from build123d import *

# Parameters (mm, degrees)
SKETCH1_R                        = 4
BOSS_EXTRUDE1_DEPTH              = 90
CHAMFER1_SIZE                    = 0.6
CUT_EXTRUDE1_START               = -1.4
SKETCH2_R                        = 4
SKETCH2_R_2                      = 3.8
CUT_EXTRUDE1_DEPTH               = 0.9
TAP_DRILL_FOR_M3_HELICOIL1_D     = 3.15
TAP_DRILL_FOR_M3_HELICOIL1_DEPTH = 6


with BuildPart() as part:
    # Sketch1 → Boss-Extrude1 (new body)
    with BuildSketch(Plane(origin=(0, 0, 0), x_dir=(1, 0, 0), z_dir=(0, 1, 0))):
        with Locations(Location((0, 0, 0), (0, 0, 90))):
            Circle(SKETCH1_R)
    extrude(amount=BOSS_EXTRUDE1_DEPTH)

    # Chamfer1
    chamfer1_edges = [part.edges().sort_by_distance(p)[0] for p in [
        (0, 0, 4),
        (0, 90, 4),
    ]]
    chamfer(chamfer1_edges, length=CHAMFER1_SIZE)

    # Sketch2 → Cut-Extrude1 (cut)
    with BuildSketch(Plane.XZ.offset(CUT_EXTRUDE1_START)):
        with Locations(Location((0, 0, 0), (0, 0, 270))):
            Circle(SKETCH2_R)
        with Locations(Location((0, 0, 0), (0, 0, 270))):
            Circle(SKETCH2_R_2, mode=Mode.SUBTRACT)
    cut_extrude1 = extrude(amount=-CUT_EXTRUDE1_DEPTH, mode=Mode.SUBTRACT)

    # Tap Drill for M3 Helicoil1
    with Locations(Plane(origin=(0, 90, 0), x_dir=(1, 0, 0), z_dir=(0, 1, 0))):
        with Locations((0, 0)):
            Hole(TAP_DRILL_FOR_M3_HELICOIL1_D / 2, depth=TAP_DRILL_FOR_M3_HELICOIL1_DEPTH)

    # Mirror1: Cut-Extrude1 across plane
    add(cut_extrude1.mirror(Plane(origin=(0, 45, 0), x_dir=(0, 0, 1), z_dir=(0, -1, 0))), mode=Mode.SUBTRACT)


solid = part.part
The model under review builds one solid part; all positions refer to its coordinate system, in mm. A direction names the side the tool comes from. Give positions to 0.01 mm unless a question says otherwise; leave off trailing zeros. Order: outer loops, then holes, each group sorted by start corner. A loop starts at its lowest first (then second) coordinate and runs counter-clockwise, first axis right, second up. Notation, with made-up numbers: (53, 49.5) -> (69, 49.5) arc R17 ccw to (69, 66.5) -> close; hole circle Ø1 at (32.25, 61.5). An arc over 180 degrees is marked (long way). Write item = value, one per line. Start each with the question number.
(1) Take a section at A-A (x = 0). Write out the cut boundary in (y, z) (3 decimals).
(2) Take a section at B-B (z = 0). Write out the cut boundary in (x, y) (3 decimals).
(3) Tool access review of faces 4 (the cylindrical face through (3.905, 0.994, 0.867)), 5 (the flat face through (0, 84, 0)), 6 (the cylindrical face through (-1.46, 88.16, -3.51)): name each direction out of +Z, -Z, +X, -X, +Y, -Y from which nothing blocks a thin tool from reaching the whole face with its end or side.
(4) For L1, parallel to Z at x = 0, y = 88.85 (3 decimals); L2, parallel to Z at x = -0.25, y = 26.5; L3, parallel to Y at x = 0.5, z = -0.5, list the stretches that pass through material, from the lowest coordinate up. Write a range as from..to.
(5) Draft analysis for pull direction Y (two halves, no side actions). For faces 1 (the cylindrical face through (-1.46, 1.84, -3.51)), 2 (the cylindrical face through (3.905, 44.402, 0.867)), 3 (the flat face through (1, 90, 2)), state which applies: +Y half, -Y half, draft (parallel to the pull), parting line (faces both ways), or undercut.
(6) Take a section at C-C (y = 19.5). Write out the cut boundary in (x, z), plus the area to 3 significant figures.
(7) For pin 1 Ø4 at (x, z) = (-2, -1) entering from -Y; pin 2 Ø1 at (y, z) = (69.5, 2.5) entering from -X; pin 3 Ø2 at (y, z) = (53, -2) entering from +X; pin 4 Ø1.5 at (x, y) = (-1, 72.5) entering from -Z, all flat-tipped, find the tip position at first contact; note any pin that passes through.
Returned:
q1.outline = (0, -3.4) -> (0.6, -4) -> (1.4, -4) -> (1.4, -3.8) -> (2.3, -3.8) -> (2.3, -4) -> (87.7, -4) -> (87.7, -3.8) -> (88.6, -3.8) -> (88.6, -4) -> (89.4, -4) -> (90, -3.4) -> (90, -1.575) -> (84, -1.575) -> (84, 1.575) -> (90, 1.575) -> (90, 3.4) -> (89.4, 4) -> (88.6, 4) -> (88.6, 3.8) -> (87.7, 3.8) -> (87.7, 4) -> (2.3, 4) -> (2.3, 3.8) -> (1.4, 3.8) -> (1.4, 4) -> (0.6, 4) -> (0, 3.4) -> close
q2.outline = (-4, 0.6) -> (-3.4, 0) -> (3.4, 0) -> (4, 0.6) -> (4, 1.4) -> (3.8, 1.4) -> (3.8, 2.3) -> (4, 2.3) -> (4, 87.7) -> (3.8, 87.7) -> (3.8, 88.6) -> (4, 88.6) -> (4, 89.4) -> (3.4, 90) -> (1.575, 90) -> (1.575, 84) -> (-1.575, 84) -> (-1.575, 90) -> (-3.4, 90) -> (-4, 89.4) -> (-4, 88.6) -> (-3.8, 88.6) -> (-3.8, 87.7) -> (-4, 87.7) -> (-4, 2.3) -> (-3.8, 2.3) -> (-3.8, 1.4) -> (-4, 1.4) -> close
q3.face_4 = +Y, -Y
q3.face_5 = +Y
q3.face_6 = none
q4.L1 = -4..-1.575, 1.575..4
q4.L2 = -3.99..3.99
q4.L3 = 0..84
q5.face_1 = undercut
q5.face_2 = draft
q5.face_3 = +Y half
q6.outline = circle Ø8 at (0, 0)
q6.area = 50.3 mm²
q7.pin_1 = 0
q7.pin_2 = -3.46
q7.pin_3 = 3.87
q7.pin_4 = -3.99
